Geometry: final body of the model. Coordinates: model frame, mm. Face numbers are marked on the shaded views. Round coordinates to 2 decimals unless told otherwise and drop trailing zeros. Write each loop counter-clockwise with the first axis right and the second up, starting at its lowest first coordinate (ties: lowest second). Pieces come first, ordered by that corner, then holes. Notation, with made-up numbers: (22, -4.75) -> (42, -4.75) arc R23 ccw to (42, 6.25) -> close; hole circle Ø8 at (20, -12). An arc over 180 degrees is marked (long way). Use one line per item in the form item = value. Start each with the question number.
1. Cut plane C-C, the plane z = -15.5. Return the cut outline in (x, y).
2. Pin query (flat end, axial travel): pin 1 Ø4.5 at (y, z) = (55, -14) entering from +X. Return the tip coordinate at first contact, or that it passes through.
3. Cut plane A-A, the plane z = -4.5. Return the cut outline in (x, y).
4. Draft query along X for the marked faces 1, 2, 3 and 4. Return one class per face: pulls with the +X half, pulls with the -X half, needs draft (parallel to the pull), parting line crosses it, or undercut.
5. Cut plane D-D, the plane y = 46. Return the cut outline in (x, z), plus the area to 3 significant figures.
6. Line query: L1, parallel to Y at x = 0.75, z = -14; L2, parallel to X at y = 39, z = -12; L3, parallel to Z at x = 59.05, y = 15. Output: solid intervals per line, ascending.
7. Cut plane B-B, the plane y = 15. Return the cut outline in (x, z).
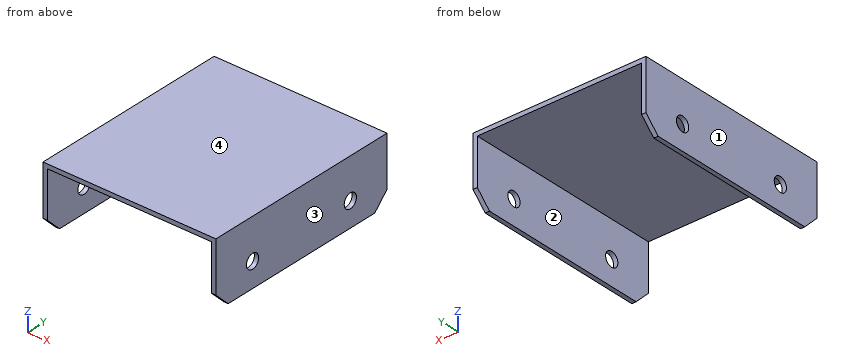
```python
from build123d import *

# Parameters (mm, degrees)
BOSS_EXTRUDE1_DEPTH = 70
SKETCH3_R           = 2.5
CUT_EXTRUDE1_DEPTH  = 60
CHAMFER1_SIZE       = 5


with BuildPart() as part:
    # Sketch1 → Boss-Extrude1 (new body)
    with BuildSketch(Plane(origin=(0, 0, 0), x_dir=(1, 0, 0), z_dir=(0, 1, 0))):
        Polygon((0, 0), (60, 0), (60, 22.5), (58.5, 22.5), (58.5, 1.5), (1.5, 1.5), (1.5, 22.5), (0, 22.5), align=None)
    extrude(amount=BOSS_EXTRUDE1_DEPTH)

    # Sketch3 → Cut-Extrude1 (cut)
    with BuildSketch(Plane(origin=(60, 0, 0), x_dir=(0, 0, -1), z_dir=(1, 0, 0))):
        with Locations((14, 55)):
            Circle(SKETCH3_R)
        with Locations(Location((14, 15, 0), (0, 0, 180))):
            Circle(SKETCH3_R)
    extrude(amount=-CUT_EXTRUDE1_DEPTH, mode=Mode.SUBTRACT)

    # Chamfer1
    chamfer1_edges = [part.edges().sort_by_distance(p)[0] for p in [
        (0.75, 0, -22.5),
        (59.25, 70, -22.5),
        (0.75, 70, -22.5),
        (59.25, 0, -22.5),
    ]]
    chamfer(chamfer1_edges, length=CHAMFER1_SIZE)


solid = part.part
```
Outcome:
q1.outline = (0, 0) -> (1.5, 0) -> (1.5, 13) -> (0, 13) -> close; (0, 17) -> (1.5, 17) -> (1.5, 53) -> (0, 53) -> close; (0, 57) -> (1.5, 57) -> (1.5, 70) -> (0, 70) -> close; (58.5, 0) -> (60, 0) -> (60, 13) -> (58.5, 13) -> close; (58.5, 17) -> (60, 17) -> (60, 53) -> (58.5, 53) -> close; (58.5, 57) -> (60, 57) -> (60, 70) -> (58.5, 70) -> close
q2.pin_1 = through
q3.outline = (0, 0) -> (1.5, 0) -> (1.5, 70) -> (0, 70) -> close; (58.5, 0) -> (60, 0) -> (60, 70) -> (58.5, 70) -> close
q4.face_1 = pulls with the -X half
q4.face_2 = undercut
q4.face_3 = pulls with the +X half
q4.face_4 = needs draft
q5.outline = (0, -22.5) -> (1.5, -22.5) -> (1.5, -1.5) -> (58.5, -1.5) -> (58.5, -22.5) -> (60, -22.5) -> (60, 0) -> (0, 0) -> close
q5.area = 153 mm^2
q6.L1 = 0 to 12.5, 17.5 to 52.5, 57.5 to 70
q6.L2 = 0 to 1.5, 58.5 to 60
q6.L3 = -22.5 to -16.5, -11.5 to 0
q7.outline = (0, -22.5) -> (1.5, -22.5) -> (1.5, -16.5) -> (0, -16.5) -> close; (0, -11.5) -> (1.5, -11.5) -> (1.5, -1.5) -> (58.5, -1.5) -> (58.5, -11.5) -> (60, -11.5) -> (60, 0) -> (0, 0) -> close; (58.5, -22.5) -> (60, -22.5) -> (60, -16.5) -> (58.5, -16.5) -> close
